Can you work these out from the model? Positions are in its coordinate system, mm. A direction names the side the tool comes from. Give positions to 0.01 mm unless a question says otherwise; leave off trailing zeros. Order: outer loops, then holes, each group sorted by start corner. A loop starts at its lowest first (then second) coordinate and runs counter-clockwise, first axis right, second up. Notation, with made-up numbers: (-28, 3.25) - (-6, 3.25) arc R27 cw to (-6, 40.25) - close; hole circle Ø3 at (-5.5, 29.5). An arc over 180 degrees is marked (long way). Write each question's results on one line, items separated by ' | '. Start each with the question number.
Autodesk Inventor part; units mm, degrees
ref_plane "Startebene" through (0, 0, 0) normal (0, 0, 1) x (1, 0, 0)
ref_plane "Endebene" through (0, 0, 104.5) normal (0, 0, 1) x (1, 0, 0)
ref_plane "YZ Plane" through (0, 0, 0) normal (1, 0, 0) x (0, 1, 0)
ref_plane "Startebene" through (0, 0, 0) normal (0, 0, 1) x (1, 0, 0)
ref_plane "Endebene" through (0, 0, 104.5) normal (0, 0, 1) x (1, 0, 0)
sketch "Skizze" plane through (0, 0, 0) normal (0, 0, 1) x (1, 0, 0)
  circle A0 centre (0, 0) radius 24
  circle A1 centre (0, 0) radius 35
  dimension "d0" = 70
  dimension "d1" = 11
extrude "Körper" add sketch "Skizze" along normal up to surface (104.5 mm away) from surface at 0
sketch "Sketch3" plane through (0, 0, 0) normal (0, 0, 1) x (1, 0, 0)
  line L0 (0, 0) -> (10, 0)
ref_plane "Work Plane3" through (0, 0, 0) normal (0, -1, 0) x (1, 0, 0)
sketch "Sketch4" plane through (0, 0, 0) normal (0, -1, 0) x (1, 0, 0)
  line L0 (-2, 0) -> (12, 0)
  line L1 (-2, 104.5) -> (12, 104.5)
  dimension "d7" = 104.5
sketch "Skizze5" plane through (0, 0, 104.5) normal (0, 0, 1) x (1, 0, 0)
  circle A0 centre (0, 0) radius 24
  line L0 (-49, 0) -> (49, 0)
  point P0 (-30, 0)
  point P1 (15, 25.9808)
  point P2 (15, -25.9808)
  dimension "d8" = 30
  dimension "d11" = 360
hole "Bohrung1" at (-30, 0, 104.5) at (15, 25.9808, 104.5) at (15, -25.9808, 104.5) direction (0, 0, -1) diameter 4 depth 20 tip angle 118
thread "Gewinde1"
thread "Gewinde2"
thread "Gewinde3"
sketch "Skizze6" plane through (0, 0, 104.5) normal (0, 0, 1) x (1, 0, 0)
  circle A0 centre (0, 0) radius 24
  circle A1 centre (0, 0) radius 35
  circle A2 centre (0, 0) radius 25
  dimension "d29" = 1
extrude "Extrusion2" cut sketch "Skizze6" against normal blind 12 contours A2
ref_plane "Arbeitsebene4" through (0, 0, 0) normal (0, 0, -1) x (-1, 0, 0)
sketch "Skizze7" plane through (0, 0, 0) normal (0, 0, -1) x (-1, 0, 0)
  circle A0 centre (0, 0) radius 24
  circle A1 centre (0, 0) radius 32
  circle A2 centre (0, 0) radius 25
  dimension "d32" = 1
extrude "Extrusion3" cut sketch "Skizze7" against normal blind 12 contours A2
equation "\"d0\" = G_H"
equation "\"d1\" = G_T"
equation "\"d2\" = G_L"
equation "\"G_H\" = 70"
equation "\"G_T\" = 11"
equation "\"G_L\" = d7"
equation "\"G_OFFSET_START\" = 0"
equation "\"G_OFFSET_END\" = 0"
equation "\"d5\" = G_OFFSET_END + B_L"
equation "\"B_L\" = 104.5"
properties part number "DIN EN 10220-2 - 57 x 5 - 100" material "Stahl, weich"
Q1. If I drill on probe 1 along Y at (x, z) = (0, 4); probe 2 along Y at (x, z) = (0, 29); probe 3 along Y at (x, z) = (15, 96.25), over which ranges is the centre line in solid material (lowest first)? Write a range as from..to.
Q2. If we section it at B-B (y = -17): Please give me the cut outline in (x, z), plus the area to 3 significant figures.
Q3. Thinking about a two-plate mould opening in Y: for faces 4 (the cylindrical face through (23.846, 7.509, 98.584)), 5 (the flat face through (-24, 8, 0)), 6 (the cylindrical face through (-28, 21, 52)), which applies, released by +Y, released by -Y, zero draft, split by the parting line, or undercut?
Q4. If we section it at D-D (z = 24): Please give me the cut outline in (x, y).
Q5. If we section it at C-C (z = 87): Please give me the cut outline in (x, y).
Q6. If we section it at A-A (x = 0): Please give me the cut outline in (y, z).
Q7. Will these pins go through, and if not, where does the flat tip stop? P1, Ø8, axis at y = 14, z = 13, coming from the +X side; P2, Ø1.5, axis at x = -14.5, z = 40, coming from the -Y side; P3, Ø15, axis at x = -10, y = -7, coming from the +Z side; P4, Ø8, axis at y = -9, z = 40.5, coming from the -X side.
Q8. Which directions (+Z, -Z, +X, -X, +Y, -Y) give clear straight access to the entire face, cutting with the end or side of a thin tool? Please do faces 1 (the cylindrical face through (-23.977, -1.055, 51.686)), 2 (the cylindrical face through (-23.846, 7.509, 5.916)), 3 (the flat face through (-9.4, 22.3, 92.5)).
Findings below:
1) probe 1: y = -35..-25, 25..35 | probe 2: y = -35..-24, 24..35 | probe 3: y = -31.62..-27.98, -23.98..-20, 20..23.98, 27.98..31.62
2) outline: (-30.59, 0) - (-18.33, 0) - (-18.33, 12) - (-16.94, 12) - (-16.94, 92.5) - (-18.33, 92.5) - (-18.33, 104.5) - (-30.59, 104.5) - close; (16.94, 12) - (18.33, 12) - (18.33, 0) - (30.59, 0) - (30.59, 104.5) - (18.33, 104.5) - (18.33, 92.5) - (16.94, 92.5) - close | area: 2,790 mm2
3) face 4: undercut | face 5: zero draft | face 6: split by the parting line
4) outline: circle Ø70 at (0, 0); hole circle Ø48 at (0, 0)
5) outline: circle Ø70 at (0, 0); hole circle Ø4 at (-30, 0); hole circle Ø48 at (0, 0); hole circle Ø4 at (15, -25.98); hole circle Ø4 at (15, 25.98)
6) outline: (-35, 0) - (-25, 0) - (-25, 12) - (-24, 12) - (-24, 92.5) - (-25, 92.5) - (-25, 104.5) - (-35, 104.5) - close; (24, 12) - (25, 12) - (25, 0) - (35, 0) - (35, 104.5) - (25, 104.5) - (25, 92.5) - (24, 92.5) - close
7) P1: stops at x = 33.54 | P2: stops at y = -32.19 | P3: passes through | P4: stops at x = -34.64
8) face 1: +Z, -Z | face 2: -Z | face 3: +Z
